Input: part model. Units: mm. Frame: model coordinates. A direction names the side the tool comes from. Coordinates: 2 decimals unless noted, no trailing zeros. Order: outer loops, then holes, each group sorted by start corner. A loop starts at its lowest first (then second) coordinate and runs counter-clockwise, first axis right, second up. Notation, with made-up numbers: (22, 61) -> (34, 61) arc R28 ccw to (34, 94) -> close; hole circle Ø2 at (88.5, -20.75). An arc over 180 degrees is marked (long way). Use one line per item in the form item = value. Start each with the question number.
1) Section query C-C on y = -15.5. Output: boundary loops of the cut face in (x, z).
2) Access query for faces 4 (the cylindrical face through (16, -7, 36)), 5 (the flat face through (17, 6.35, 37)), 6 (the flat face through (-6.35, -17, 36)). Directions: +Z, -Z, +X, -X, +Y, -Y. A direction counts if a zero-diameter tool reaches every point of the face in a straight line with its end or side. Return the directions, or none.
3) Section query A-A on z = 55. Count the separate pieces of the cut face and the enclosed holes in it, then the cut area to 3 significant figures.
4) Pin query (flat end, axial travel): pin 1 (4 mm diameter, centred on x = 1, y = -14, fed in from -Z); pin 2 (0.8 mm diameter, centred on y = -17, z = 43, fed in from -X); pin 3 (1.9 mm diameter, centred on x = 17, z = 26.5, fed in from +Y); pin 4 (0.8 mm diameter, centred on x = -17, z = 47, fed in from -Y). Return the tip coordinate at first contact, or that it passes through.
5) Section query B-B on x = 0. Output: boundary loops of the cut face in (y, z).
6) Section query D-D on x = -10. Output: boundary loops of the cut face in (y, z), then the cut area to 3 significant figures.
7) Ray query, line 1 along X through (y, z) = (-17, 40.5); line 2 along X through (y, z) = (-9.5, 6.5); line 3 along Y through (x, z) = (8, 66). Return the intervals inside material, ascending.
8) Draft query along Y for faces 1 (the cylindrical face through (17.597, -7.296, 35.688)), 2 (the cylindrical face through (-17.64, 0.14, 66.04)), 3 (the flat face through (6.35, 17, 36)). Return one class per face: pulls with the +Y half, pulls with the -Y half, needs draft (parallel to the pull), parting line crosses it, or undercut.
from build123d import *

# Parameters (mm, degrees)
F0_R            = 19.05
F0_R_2          = 17.4625
F1_DEPTH        = 72.39
F3_DEPTH        = 25.4
F3_COPIES_COUNT = 4


# Not quite as in the source:
# - a pattern or mirror of a feature is missing from the dataset's text; its kind, count and spacing are read off the source's solid


with BuildPart() as f1:
    # F0 (on Top) → F1 (new body)
    with BuildSketch(Plane.XY):
        Circle(F0_R)
        Circle(F0_R_2, mode=Mode.SUBTRACT)
    extrude(amount=F1_DEPTH)

    # F2 (on Front) → F3 (cut)
    with BuildSketch(Plane.XZ):
        with BuildLine():
            Line((-6.35, 59.69), (-6.35, 12.7))
            ThreePointArc((-6.35, 12.7), (0, 6.35), (6.35, 12.7))
            Line((6.35, 12.7), (6.35, 59.69))
            ThreePointArc((6.35, 59.69), (0, 66.04), (-6.35, 59.69))
        make_face()
    f3 = extrude(amount=-F3_DEPTH, mode=Mode.SUBTRACT)

    # F3_copies: F3 ×4 about axis
    f3_copies_axis = Axis((0, 0, 0), (0, 0, 1))
    for i in range(1, F3_COPIES_COUNT):
        add(f3.rotate(f3_copies_axis, i * 360 / F3_COPIES_COUNT), mode=Mode.SUBTRACT)


solid = f1.part
Answers below:
q1.outline = (-11.07, 0) -> (-8.04, 0) -> (-8.04, 72.39) -> (-11.07, 72.39) -> close; (8.04, 0) -> (11.07, 0) -> (11.07, 72.39) -> (8.04, 72.39) -> close
q2.face_4 = +Z, -Z
q2.face_5 = +X, -X
q2.face_6 = +Y, -Y
q3.separate_pieces = 4
q3.enclosed_holes = 0
q3.area = 99.7 mm^2
q4.pin_1 = through
q4.pin_2 = -9.35
q4.pin_3 = 10.26
q4.pin_4 = -9.35
q5.outline = (-19.05, 0) -> (-17.46, 0) -> (-17.46, 6.35) -> (-19.05, 6.35) -> close; (-19.05, 66.04) -> (-17.46, 66.04) -> (-17.46, 72.39) -> (-19.05, 72.39) -> close; (17.46, 0) -> (19.05, 0) -> (19.05, 6.35) -> (17.46, 6.35) -> close; (17.46, 66.04) -> (19.05, 66.04) -> (19.05, 72.39) -> (17.46, 72.39) -> close
q6.outline = (-16.21, 0) -> (-14.32, 0) -> (-14.32, 72.39) -> (-16.21, 72.39) -> close; (14.32, 0) -> (16.21, 0) -> (16.21, 72.39) -> (14.32, 72.39) -> close
q6.area = 275 mm^2
q7.line_1 = -8.6 to -6.35, 6.35 to 8.6
q7.line_2 = -16.51 to -14.65, 14.65 to 16.51
q7.line_3 = -17.29 to -15.52, 15.52 to 17.29
q8.face_1 = parting line crosses it
q8.face_2 = undercut
q8.face_3 = needs draft
